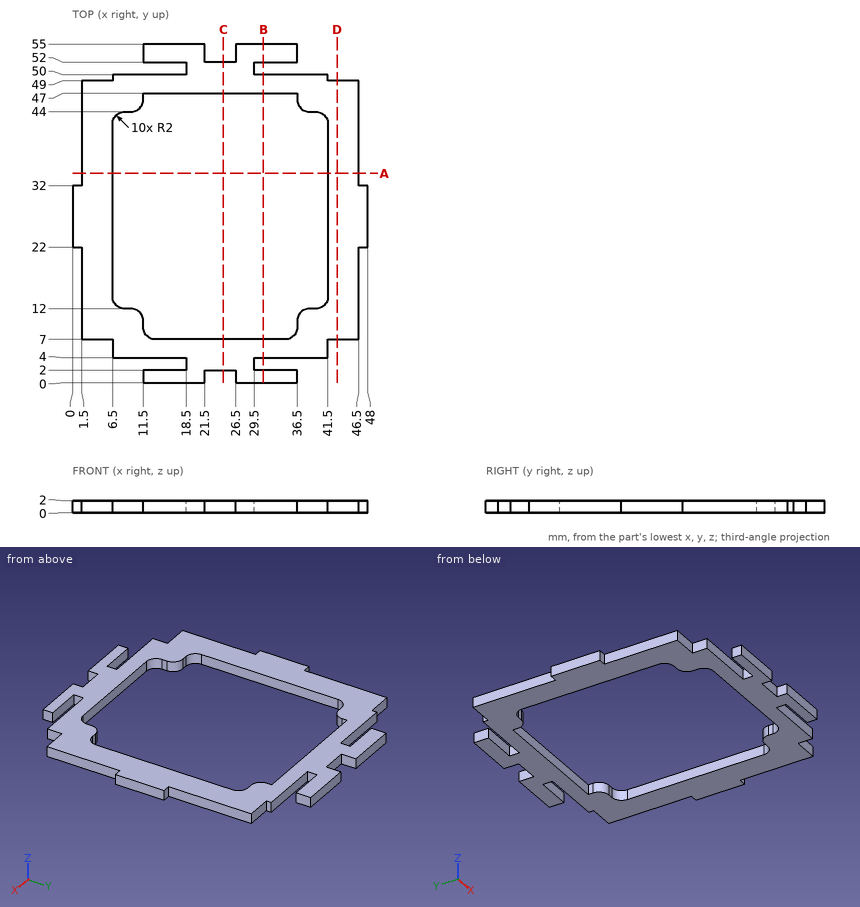
The figure shows three views and two pictorial views of one solid part (mm, origin at its lowest corner). Answer the questions. Coordinates: 2 decimals unless noted, no trailing zeros. Loops run counter-clockwise (first coordinate to the right, second up) from the corner with the lowest first, then second, coordinate; pieces in that order, holes last.
1) Find section A-A on y = 34. Write down the section's boundary in (x, z).
2) Find section B-B on x = 31. Write down the section's boundary in (y, z), then the cut area to 3 significant figures.
3) Find section C-C on x = 24.5. Write down the section's boundary in (y, z).
4) Find the intervals of material crossed by L1, parallel to Y at x = 31.5, z = 1.35; L2, parallel to X at y = 19, z = 0.9; L3, parallel to X at y = 31, z = 0.8, in increasing order.
5) Find section D-D on x = 43. Write down the section's boundary in (y, z), then the cut area to 3 significant figures.
6) Flat-ended cylindrical pins translate along their axes: pin 1 Ø0.6 at (x, z) = (37.5, 1.5) entering from +Y; pin 2 Ø1.2 at (x, z) = (47.5, 0.5) entering from +Y; pin 3 Ø1 at (y, z) = (34, 1) entering from -X. Find the tip coordinate at first contact, or state that the pin passes through.
Values:
1. outline: (1.5, 0) - (6.5, 0) - (6.5, 2) - (1.5, 2) - close; (41.5, 0) - (46.5, 0) - (46.5, 2) - (41.5, 2) - close
2. outline: (0, 0) - (2, 0) - (2, 2) - (0, 2) - close; (4, 0) - (7, 0) - (7, 2) - (4, 2) - close; (47, 0) - (50, 0) - (50, 2) - (47, 2) - close; (52, 0) - (55, 0) - (55, 2) - (52, 2) - close
2. area: 22.0 mm2
3. outline: (2, 0) - (7, 0) - (7, 2) - (2, 2) - close; (47, 0) - (52, 0) - (52, 2) - (47, 2) - close
4. L1: y = 0 to 2, 4 to 7, 47 to 50, 52 to 55
4. L2: x = 1.5 to 6.5, 41.5 to 46.5
4. L3: x = 0 to 6.5, 41.5 to 48
5. outline: (7, 0) - (49, 0) - (49, 2) - (7, 2) - close
5. area: 84.0 mm2
6. pin 1: stops at y = 50
6. pin 2: stops at y = 32
6. pin 3: stops at x = 1.5
